The model under review builds one solid part; all positions refer to its coordinate system, in mm. A direction names the side the tool comes from. Give positions to 0.01 mm unless a question says otherwise; leave off trailing zeros. Loops run counter-clockwise (first coordinate to the right, second up) from the corner with the lowest first, then second, coordinate; pieces in that order, holes last. Notation, with made-up numbers: M -4.75,29.5 L 18.25,29.5 A12 ccw 18.25,50.5 Z; hole C 42,-19 d4. An arc over 180 degrees is marked long. Return JSON: item names as keys, results as strings. Group by question number.
Autodesk Inventor part; units mm, degrees
ref_plane "YZ Plane" through (0, 0, 0) normal (1, 0, 0) x (0, 1, 0)
ref_plane "XZ Plane" through (0, 0, 0) normal (0, 1, 0) x (-1, 0, 0)
ref_plane "XY Plane" through (0, 0, 0) normal (0, 0, 1) x (1, 0, 0)
ref_plane "Work Plane1" through (0, 30, 0) normal (0, 0, 1) x (1, 0, 0)
sketch "Sketch1" plane through (0, 30, 0) normal (0, 0, 1) x (1, 0, 0)
  line L0 (0, 6) -> (12, 6)
  line L1 (0, 0) -> (0, 6)
  line L2 (12, 0) -> (0, 0)
  line L3 (12, 0) -> (12, 6)
  line L4 (28, -6) -> (28, -18)
  line L5 (22, -6) -> (28, -6)
  line L6 (22, -18) -> (22, -6)
  line L7 (22, -18) -> (28, -18)
  line L8 (0, -24) -> (12, -24)
  line L9 (0, -30) -> (0, -24)
  line L10 (12, -30) -> (0, -30)
  line L11 (12, -30) -> (12, -24)
  line L12 (-10, -6) -> (-10, -18)
  line L13 (-16, -6) -> (-10, -6)
  line L14 (-16, -18) -> (-16, -6)
  line L15 (-16, -18) -> (-10, -18)
  line L16 (-10, 0) -> (0, 0)
  line L17 (12, 0) -> (22, 0)
  line L18 (22, 6) -> (22, -6)
  line L19 (22, -18) -> (22, -30)
  line L20 (12, -24) -> (22, -24)
  line L21 (0, -24) -> (-10, -24)
  line L22 (-10, -30) -> (-10, -18)
  line L23 (-10, -6) -> (-10, 6)
extrude "Extrusion1" add sketch "Sketch1" along normal blind 6
equation "\"BendRadius\" = Thickness"
equation "\"BendReliefWidth\" = Thickness"
equation "\"BendReliefDepth\" = 0.5 * Thickness"
equation "\"CornerReliefSize\" = 4 * Thickness"
equation "\"MinimumRemnant\" = 2 * Thickness"
equation "\"TransitionRadius\" = BendRadius"
equation "\"JacobiRadiusSize\" = Thickness"
equation "\"GapSize\" = Thickness"
properties part number "onderkantBovenkant knoppendoosje" material "Wood (Birch)"
(1) For probe 1 along X at (y, z) = (11, 1.65); probe 2 along Y at (x, z) = (20.5, 5.3); probe 3 along Y at (x, z) = (24.5, 3.65), list the stretches that pass through material, from the lowest coordinate up.
(2) Add section A-A (z = 4.1). Write out the cut boundary in (x, y), and give its area (3 significant figures).
(3) For faces 1 (the flat face through (-5, 6, 3)), 2 (the flat face through (6, 0, 3)), 3 (the flat face through (22, 27, 3)), 4 (the flat face through (0, 33, 3)), 5 (the flat face through (12, 3, 3)), list the 3-axis set-ups (+Z, -Z, +X, -X, +Y, -Y) from which the entire face can be reached by the end or side of a thin tool; tool diameter is ignored.
(4) For pin 1 (2 mm diameter, centred on x = -4, z = 1, fed in from -Y); pin 2 (3 mm diameter, centred on y = 3.5, z = 1.5, fed in from +X); pin 3 (1.8 mm diameter, centred on x = 19, z = 1.5, fed in from +Y), all flat-tipped, find the tip position at first contact; note any pin that passes through.
(5) Add section C-C (x = -5.5). Write out the cut boundary in (y, z), and give its area (3 significant figures).
(6) Add section B-B (y = 31). Write out the cut boundary in (x, z), and give its area (3 significant figures).
Verdict:
{
 "1": {"probe 1": "x = -10 to 22", "probe 2": "y = 6 to 30", "probe 3": "y = 12 to 24"},
 "2": {"outline": "M -16,12 L -10,12 L -10,6 L 0,6 L 0,0 L 12,0 L 12,6 L 22,6 L 22,12 L 28,12 L 28,24 L 22,24 L 22,30 L 12,30 L 12,36 L 0,36 L 0,30 L -10,30 L -10,24 L -16,24 Z", "area": "1,060 mm²"},
 "3": {"face 1": "+Z, -Z, -X, -Y", "face 2": "+Z, -Z, +X, -X, -Y", "face 3": "+Z, -Z, +X, +Y", "face 4": "+Z, -Z, -X, +Y", "face 5": "+Z, -Z, +X, -Y"},
 "4": {"pin 1": "stops at y = 6", "pin 2": "stops at x = 12", "pin 3": "stops at y = 30"},
 "5": {"outline": "M 6,0 L 30,0 L 30,6 L 6,6 Z", "area": "144 mm²"},
 "6": {"outline": "M 0,0 L 12,0 L 12,6 L 0,6 Z", "area": "72.0 mm²"}
}
